Read the model definition and answer for the solid it produces. Units are mm, in the model's axes. Face numbers are marked on the shaded views. A direction names the side the tool comes from. Give positions to 0.01 mm unless a question says otherwise; leave off trailing zeros. Loops run counter-clockwise (first coordinate to the right, second up) from the corner with the lowest first, then second, coordinate; pieces in that order, holes last. Notation, with made-up numbers: (70, 42) - (116, 42) arc R12 cw to (116, 62) - close; hole circle Ø3 at (44, 28.5). An arc over 180 degrees is marked (long way). Put each result on its own line as item: value. Start each with the question number.
1. A cutting plane is placed at C-C, the plane x = -46. Determine the outline of the cut face in (y, z).
2. For a pull along Y with two mould halves and no side action, classify the marked faces 3, 4 and 5 as released by +Y, released by -Y, zero draft, split by the parting line, or undercut.
3. Given pin 1 Ø4 at (x, y) = (-63.5, -10) entering from +Z; pin 2 Ø1.5 at (x, z) = (-59.5, 3.5) entering from -Y; pin 3 Ø22 at (x, y) = (0, 0) entering from -Z; pin 4 Ø1 at (x, z) = (-47.5, 1.5) entering from -Y, each flat-ended and moving along its own axis, determine where each tip first touches the part or whether it passes through.
4. A cutting plane is placed at D-D, the plane y = -28. Determine the outline of the cut face in (x, z), plus the area to 3 significant figures.
5. A cutting plane is placed at B-B, the plane y = 11.5. Determine the outline of the cut face in (x, z), plus the area to 3 significant figures.
6. Consider L1, parallel to X at y = 4.5, z = 3.25; L2, parallel to Y at x = -61, z = 0.5; L3, parallel to Y at x = -48, z = 4. Determine where each line is inside the solid, lowest interval first. Write a range as from..to.
7. A cutting plane is placed at A-A, the plane z = 5. Determine the outline of the cut face in (x, y).
8. For the marked faces 1 and 2, determine the directions among +Z, -Z, +X, -X, +Y, -Y from which every point of the face is accessible in a straight line to the end or side of a thin tool.
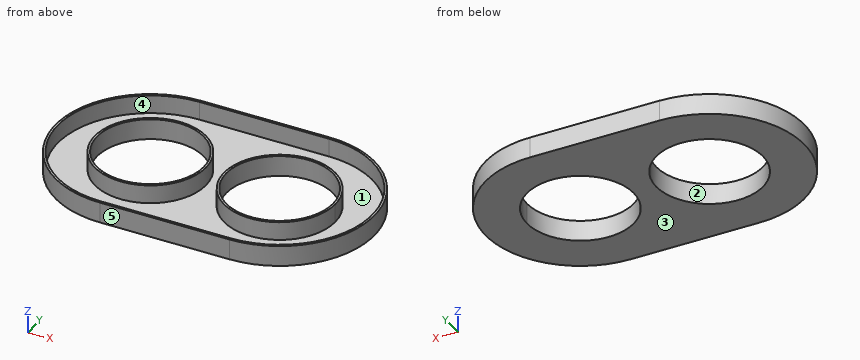
```python
from build123d import *

# Parameters (mm, degrees)
F0_R     = 19.05
F1_DEPTH = 6.35
F2_T     = 0.762


with BuildPart() as f1:
    # F0 (on Top) → F1 (new body)
    with BuildSketch(Plane.XY):
        with BuildLine():
            Line((0, 31.75), (-44.2468, 31.75))
            ThreePointArc((-44.2468, 31.75), (-75.9968, 0), (-44.2468, -31.75))
            Line((-44.2468, -31.75), (0, -31.75))
            ThreePointArc((0, -31.75), (31.75, 0), (0, 31.75))
        make_face()
        with Locations((-44.2468, 0)):
            Circle(F0_R, mode=Mode.SUBTRACT)
        with BuildLine():
            ThreePointArc((-14.8329292767, -11.9535228729), (-6.3377913061, 17.9648240003), (19.05, 0))
            ThreePointArc((19.05, 0), (6.3377913061, -17.9648240003), (-14.8329292767, -11.9535228729))
        make_face(mode=Mode.SUBTRACT)
    extrude(amount=F1_DEPTH)

    # F2
    f2_openings = [f1.faces().sort_by_distance(p)[0] for p in [
        (-22.1234, 0, 6.35),
    ]]
    offset(amount=F2_T, openings=f2_openings, kind=Kind.INTERSECTION)


solid = f1.part
```
Return value:
1. outline: (-32.46, -0.76) - (-18.2, -0.76) - (-18.2, 6.35) - (-18.97, 6.35) - (-18.97, 0) - (-31.7, 0) - (-31.7, 6.35) - (-32.46, 6.35) - close; (18.2, -0.76) - (32.46, -0.76) - (32.46, 6.35) - (31.7, 6.35) - (31.7, 0) - (18.97, 0) - (18.97, 6.35) - (18.2, 6.35) - close
2. face 3: zero draft
2. face 4: undercut
2. face 5: released by -Y
3. pin 1: stops at z = 0
3. pin 2: stops at y = -29.1
3. pin 3: passes through
3. pin 4: stops at y = -32.4
4. outline: (-60.77, -0.76) - (16.52, -0.76) - (16.52, 6.35) - (14.97, 6.35) - (14.97, 0) - (-59.22, 0) - (-59.22, 6.35) - (-60.77, 6.35) - close
4. area: 78.6 mm2
5. outline: (-74.66, -0.76) - (-58.47, -0.76) - (-58.47, 6.35) - (-59.43, 6.35) - (-59.43, 0) - (-73.84, 0) - (-73.84, 6.35) - (-74.66, 6.35) - close; (-30.03, -0.76) - (-14.22, -0.76) - (-14.22, 6.35) - (-15.19, 6.35) - (-15.19, 0) - (-29.06, 0) - (-29.06, 6.35) - (-30.03, 6.35) - close; (14.22, -0.76) - (30.41, -0.76) - (30.41, 6.35) - (29.59, 6.35) - (29.59, 0) - (15.19, 0) - (15.19, 6.35) - (14.22, 6.35) - close
5. area: 71.7 mm2
6. L1: x = -76.45..-75.68, -62.76..-61.97, -26.52..-25.74, -18.51..-17.73, 17.73..18.51, 31.43..32.2
6. L2: y = -27.86..-26.97, -9.07..-7.33, 7.33..9.07, 26.97..27.86
6. L3: y = -32.29..-31.53, -18.68..-17.9, 17.9..18.68, 31.53..32.29
7. outline: circle Ø38.1 at (-44.25, 0); (-44.25, -32.51) - (0, -32.51) arc R32.51 ccw to (0, 32.51) - (-44.25, 32.51) arc R32.51 ccw to start; circle Ø38.1 at (0, 0); hole circle Ø36.58 at (-44.25, 0); hole (-44.25, -31.75) - (0, -31.75) arc R31.75 ccw to (0, 31.75) - (-44.25, 31.75) arc R31.75 ccw to start; hole circle Ø36.58 at (0, 0)
8. face 1: +Z
8. face 2: +Z, -Z
